Design review of the part shown in the three views and the two pictorial views. Dimensions are in mm from the part's minimum x, y and z. A direction names the side the tool comes from. Round coordinates to 2 decimals unless told otherwise and drop trailing zeros. Order: outer loops, then holes, each group sorted by start corner. A loop starts at its lowest first (then second) coordinate and runs counter-clockwise, first axis right, second up.
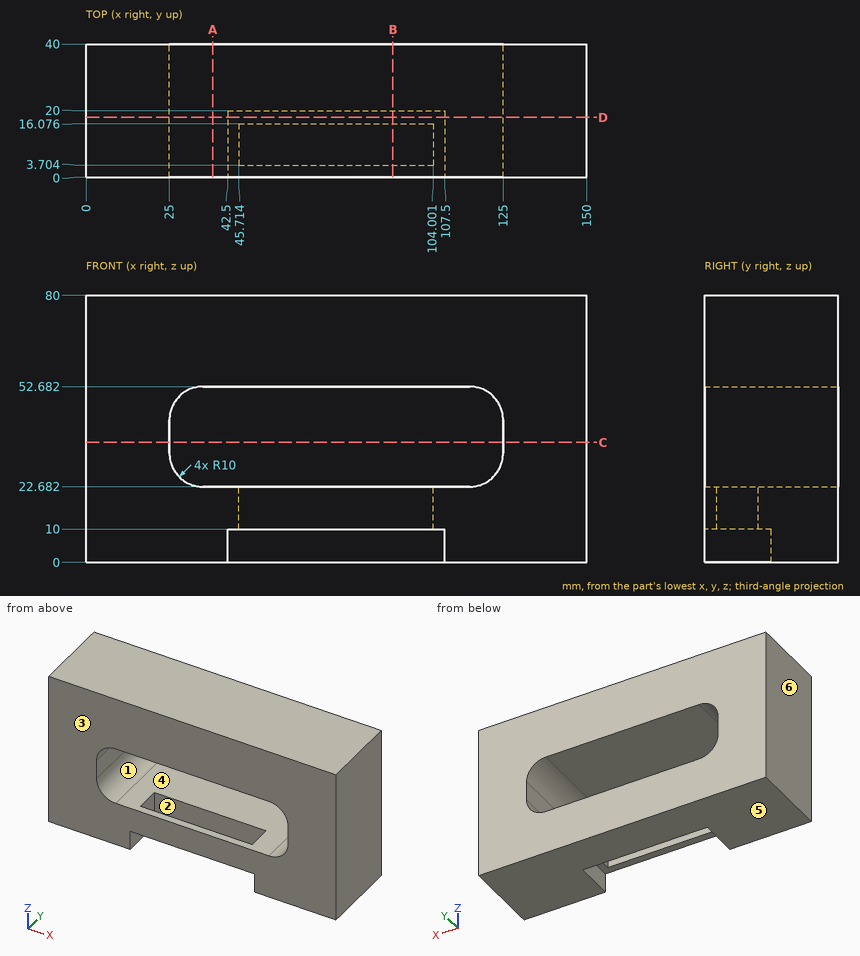
1) Take a section at B-B on x = 92. Give the boundary of the cut face in (y, z).
Results:
outline: (0, 10) - (3.7, 10) - (3.7, 22.68) - (0, 22.68) - close; (0, 52.68) - (40, 52.68) - (40, 80) - (0, 80) - close; (16.08, 10) - (20, 10) - (20, 0) - (40, 0) - (40, 22.68) - (16.08, 22.68) - close
2) Clearance check with a flat-ended pin moving along its axis: P1, Ø22, axis at x = 79, y = 7, coming from the -Z side. State where the tip first meets the part, or that it passes through.
Results:
P1: stops at z = 10
3) The part is to be moulded in two halves that separate along Z. For the marked faces 4, 5 and 6, say which applies: released by +Z, released by -Z, zero draft, split by the parting line, or undercut.
Results:
face 4: undercut
face 5: released by -Z
face 6: zero draft
4) Take a section at D-D on y = 18. Give the boundary of the cut face in (x, z), plus the area to 3 significant figures.
Results:
outline: (0, 0) - (42.5, 0) - (42.5, 10) - (107.5, 10) - (107.5, 0) - (150, 0) - (150, 80) - (0, 80) - close; hole (25, 32.68) arc R10 ccw to (35, 22.68) - (115, 22.68) arc R10 ccw to (125, 32.68) - (125, 42.68) arc R10 ccw to (115, 52.68) - (35, 52.68) arc R10 ccw to (25, 42.68) - close
area: 8,440 mm2
5) Take a section at A-A on x = 38. Give the boundary of the cut face in (y, z).
Results:
outline: (0, 0) - (40, 0) - (40, 22.68) - (0, 22.68) - close; (0, 52.68) - (40, 52.68) - (40, 80) - (0, 80) - close
6) For the marked faces 1, 2 and 3, list the 3-axis set-ups (+Z, -Z, +X, -X, +Y, -Y) from which the entire face can be reached by the end or side of a thin tool; tool diameter is ignored.
Results:
face 1: +Y, -Y
face 2: -Z
face 3: +Z, -Z, +X, -X, -Y
7) Take a section at C-C on z = 36. Give the boundary of the cut face in (x, y), plus the area to 3 significant figures.
Results:
outline: (0, 0) - (25, 0) - (25, 40) - (0, 40) - close; (125, 0) - (150, 0) - (150, 40) - (125, 40) - close
area: 2,000 mm2
8) To check wall thickness, follow line 1 along X through (y, z) = (5, 33); line 2 along X through (y, z) = (7, 14); line 3 along Y through (x, z) = (85, 12). State the ranges of each line that lie inside material, in increasing order.
Results:
line 1: x = 0 to 25, 125 to 150
line 2: x = 0 to 45.71, 104 to 150
line 3: y = 0 to 3.7, 16.08 to 40
